Here's how the part is built. I have some questions about the finished solid (model axes, mm). Face numbers are marked on the shaded views. A direction names the side the tool comes from. Give positions to 0.01 mm unless a question says otherwise; leave off trailing zeros. Loops run counter-clockwise (first coordinate to the right, second up) from the corner with the lowest first, then second, coordinate; pieces in that order, holes last.
Q1. Suppose I cut it at D-D (x = 394.5). List the corners of the cut face in (y, z) for me.
Q2. Thinking about a two-plate mould opening in X: for the marked faces 1, 2 and 3, which applies, pulls with the +X half, pulls with the -X half, needs draft (parallel to the pull), parting line crosses it, or undercut?
Q3. Suppose I cut it at C-C (x = 772). List the corners of the cut face in (y, z) for me, and give its area (3 significant figures).
Q4. For the marked faces 4, 5, 6 and 7, which set-ups out of +Z, -Z, +X, -X, +Y, -Y let a thin tool reach every point of the face, with its end or its side?
Q5. I need wall thicknesses on probe 1 along X at (y, z) = (69, -108); probe 2 along X at (y, z) = (102, -73); probe 3 along X at (y, z) = (178, 211). Which ranges of each line are inside material? Lowest first, please.
Q6. I'm going to push flat-ended pins straight in: P1, Ø12, axis at y = 184, z = -218.5, coming from the +X side; P2, Ø8, axis at x = 131.5, z = 23, coming from the +Y side; P3, Ø10, axis at y = 65.5, z = 253.5, coming from the -X side. Where does each tip first touch, or does it pass through?
```python
from build123d import *

# Parameters (mm, degrees)
F2_SIZE = 25.4


with BuildPart() as f1:
    # F0 (on Front) → F1 (revolve)
    with BuildSketch(Plane.XZ):
        Polygon((0, 177.8), (0, 0), (863.6, 0), (863.6, 172.44786), (787.4, 172.44786), (787.4, 107.95), (685.8, 107.95), (685.8, 203.2), (609.6, 203.2), (609.6, 127), (533.4, 127), (533.4, 203.2), (457.2, 203.2), (457.2, 330.2), (381, 330.2), (381, 177.8), align=None)
    revolve(axis=Axis((431.8, 0, 0), (1, 0, 0)))

    # F2
    f2_edges = [f1.edges().sort_by_distance(p)[0] for p in [
        (863.6, 0, -172.44786),
    ]]
    chamfer(f2_edges, length=F2_SIZE)


solid = f1.part
```
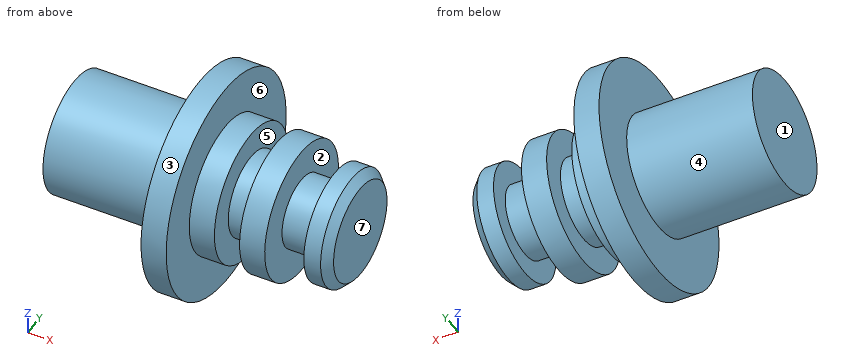
Solutions:
1. outline: circle Ø660.4 at (0, 0)
2. face 1: pulls with the -X half
2. face 2: undercut
2. face 3: needs draft
3. outline: circle Ø215.9 at (0, 0)
3. area: 36,600 mm2
4. face 4: -X
4. face 5: none
4. face 6: +X
4. face 7: +Z, -Z, +X, +Y, -Y
5. probe 1: x = 0 to 533.4, 609.6 to 685.8, 787.4 to 863.6
5. probe 2: x = 0 to 685.8, 787.4 to 863.6
5. probe 3: x = 381 to 457.2
6. P1: stops at x = 457.2
6. P2: stops at y = 176.78
6. P3: stops at x = 381
